```python
from build123d import *

# Parameters (mm, degrees)
CUT_EXTRUDE1_REACH = 69.967
SKETCH3_R          = 11
SKETCH4_R          = 16
CUT_EXTRUDE2_DEPTH = 10


with BuildPart() as part:
    # Sketch2 → Revolve1 (revolve)
    with BuildSketch(Plane.XY, mode=Mode.PRIVATE) as revolve1_sk:
        Polygon((10.935942394, 19), (-2.064057606, 19), (-2.064057606, 0), (-8.495542791, -6.431485186), (-20.464057606, -6.431485186), (-20.464057606, 0), (-25.464057606, 0), (-25.464057606, -9.462439506), (-21.464057606, -13.462439506), (10.935942394, -13.462439506), align=None)
    revolve(revolve1_sk.sketch.rotate(Axis((10.935942394, -13.462439506, 0), (0, 1, 0)), 180), axis=Axis((10.935942394, -13.462439506, 0), (0, 1, 0)))

    # Sketch3 → Cut-Extrude1 (cut, up to next)
    with BuildSketch(Plane(origin=(0, 19, 0), x_dir=(1, 0, 0), z_dir=(0, 1, 0)), mode=Mode.PRIVATE) as cut_extrude1_sk1:
        with Locations(Location((10.935942394, 0, 0), (0, 0, 180))):
            Circle(SKETCH3_R)
    cut_extrude1_tool1 = extrude(cut_extrude1_sk1.sketch, amount=-CUT_EXTRUDE1_REACH, mode=Mode.PRIVATE) & part.part
    add(cut_extrude1_tool1.solids().sort_by_distance((10.935942, 19, 0))[0], mode=Mode.SUBTRACT)

    # Sketch4 → Cut-Extrude2 (cut)
    with BuildSketch(Plane.XZ.offset(13.462439506)):
        with Locations((10.935942394, 36.4)):
            Circle(SKETCH4_R)
        with Locations((45.554399587, 11.248218595)):
            Circle(SKETCH4_R)
        with Locations((32.331325578, -29.448218595)):
            Circle(SKETCH4_R)
        with Locations((-10.459440789, -29.448218595)):
            Circle(SKETCH4_R)
        with Locations((-23.682514799, 11.248218595)):
            Circle(SKETCH4_R)
    extrude(amount=-CUT_EXTRUDE2_DEPTH, mode=Mode.SUBTRACT)


solid = part.part
```
The model under review builds one solid part; all positions refer to its coordinate system, in mm. A direction names the side the tool comes from. Give positions to 0.01 mm unless a question says otherwise; leave off trailing zeros. Write each loop counter-clockwise with the first axis right and the second up, starting at its lowest first coordinate (ties: lowest second). Pieces come first, ordered by that corner, then holes. Notation, with made-up numbers: (69.5, -15) -> (89.5, -15) arc R18 cw to (89.5, 2) -> close; hole circle Ø1 at (56, 13). An arc over 180 degrees is marked (long way). Put each result on its own line as item: value.
(1) We need section C-C, the plane z = -25. Give the boundary of the cut face in (x, y).
Results are:
outline: (-15.52, -3.46) -> (-8.06, -3.46) -> (-8.06, 0) -> (-15.52, 0) -> close; (4.91, -13.46) -> (16.96, -13.46) -> (16.96, -6.43) -> (4.91, -6.43) -> close; (29.93, -3.46) -> (37.39, -3.46) -> (37.39, 0) -> (29.93, 0) -> close
(2) We need section A-A, the plane y = -11. Give the boundary of the cut face in (x, z), and give its area (3 significant figures).
Results are:
outline: (-23.6, -4.75) arc R34.86 ccw to (-19.8, -16.46) arc R16 cw to (4.78, -34.32) arc R34.86 ccw to (17.09, -34.32) arc R16 cw to (41.67, -16.46) arc R34.86 ccw to (45.47, -4.75) arc R16 cw to (36.08, 24.14) arc R34.86 ccw to (26.13, 31.38) arc R16 cw to (-4.26, 31.38) arc R34.86 ccw to (-14.21, 24.14) arc R16 cw to start; hole circle Ø22 at (10.94, 0)
area: 1,860 mm²
(3) We need section D-D, the plane y = 5.5. Give the boundary of the cut face in (x, z), and give its area (3 significant figures).
Results are:
outline: circle Ø26 at (10.94, 0); hole circle Ø22 at (10.94, 0)
area: 151 mm²
(4) The part is to be moulded in two halves that separate along X. For faces 4 (the flat face through (22, 19, -3)), 5 (the cylindrical face through (23.336, 9.367, -3.905)), 6 (the cylindrical face through (10.634, -9.644, 20.403)), 7 (the conical face through (-21.726, -11.49, -10.706)), say which applies: pulls with the +X half, pulls with the -X half, needs draft (parallel to the pull), parting line crosses it, or undercut.
Results are:
face 4: needs draft
face 5: parting line crosses it
face 6: undercut
face 7: pulls with the -X half
(5) Tool access review of faces 1 (the flat face through (11, -3.462, 32)), 2 (the flat face through (10, -13.462, 12)), 3 (the cylindrical face through (40.886, -2.456, -9.432)): name each direction out of +Z, -Z, +X, -X, +Y, -Y from which nothing blocks a thin tool from reaching the whole face with its end or side.
Results are:
face 1: +Z, -Y
face 2: +Z, -Z, +X, -X, -Y
face 3: +Y
(6) We need section B-B, the plane z = 0. Give the boundary of the cut face in (x, y).
Results are:
outline: (-25.46, -3.46) -> (-20.46, -3.46) -> (-20.46, 0) -> (-25.46, 0) -> close; (-12.3, -13.46) -> (-0.06, -13.46) -> (-0.06, 19) -> (-2.06, 19) -> (-2.06, 0) -> (-8.5, -6.43) -> (-12.3, -6.43) -> close; (21.94, -13.46) -> (34.18, -13.46) -> (34.18, -6.43) -> (30.37, -6.43) -> (23.94, 0) -> (23.94, 19) -> (21.94, 19) -> close; (42.34, -3.46) -> (47.34, -3.46) -> (47.34, 0) -> (42.34, 0) -> close
(7) For pin 1 Ø1.5 at (x, y) = (-1.5, -9.5) entering from -Z; pin 2 Ø8 at (y, z) = (13.5, -1) entering from -X; pin 3 Ø10 at (y, z) = (-8, -23) entering from +X; pin 4 Ø5 at (y, z) = (9, 17.5) entering from -X, all flat-tipped, find the tip position at first contact; note any pin that passes through.
Results are:
pin 1: z = -16.73
pin 2: x = -2.06
pin 3: x = 40.74
pin 4: through
(8) To check wall thickness, follow probe 1 along Z at (x, y) = (-1, -2); probe 2 along Y at (x, z) = (44, 10); probe 3 along Y at (x, z) = (-8.5, 20). State the ranges of each line that lie inside material, in increasing order. Write a range as from..to.
Results are:
probe 1: -34.39..-29.04, -9.08..9.08, 29.04..34.39
probe 2: -3.46..0
probe 3: -13.46..-6.43
